Can you work these out from the model? Positions are in its coordinate system, mm. A direction names the side the tool comes from. Give positions to 0.01 mm unless a question says otherwise; leave off trailing zeros. Write each loop counter-clockwise with the first axis right and the second up, starting at its lowest first coordinate (ties: lowest second). Pieces come first, ordered by that corner, then holes.
1. If I drill on probe 1 along X at (y, z) = (20, -157); probe 2 along Y at (x, z) = (256.5, -42.5), over which ranges is the centre line in solid material (lowest first)?
2. Suppose I cut it at C-C (x = 97.5). Please give me the cut outline in (y, z), and give its area (3 significant figures).
3. On a 3-axis mill with a long thin cutter (end or side, diameter ignored), from which of +Z, -Z, +X, -X, +Y, -Y can I reach the whole of each face in a straight line? I mean faces 4 (the flat face through (-350, 30, 4)), 5 (the flat face through (-353.062, 23, 4)). Say none if no direction works.
4. Suppose I cut it at A-A (y = 12). Please give me the cut outline in (x, z).
5. I'm going to push a flat-ended pin straight in: pin 1 (8 mm diameter, centred on x = -246.5, z = -83, fed in from +Y). Where does the tip first touch, or does it pass through?
6. Thinking about a two-plate mould opening in X: for faces 1 (the flat face through (-5, -15, 4)), 2 (the flat face through (353.062, 22, 4)), 3 (the flat face through (5, 0, 4)), which applies, pulls with the +X half, pulls with the -X half, needs draft (parallel to the pull), parting line crosses it, or undercut?
7. Suppose I cut it at B-B (z = -174). Please give me the cut outline in (x, y), and give its area (3 significant figures).
```python
from build123d import *

# Parameters (mm, degrees)
SALIENTE_EXTRUIR1_DEPTH = 300


with BuildPart() as part:
    # Croquis1 → Saliente-Extruir1 (new, symmetric)
    with BuildSketch(Plane.XY):
        Polygon((0, -15), (0, 0), (-350, 0), (-350, 60), (-353.0625, 60), (-353.0625, -15), align=None)
        Polygon((350, 60), (350, 0), (0, 0), (0, -15), (353.0625, -15), (353.0625, 60), align=None)
    extrude(amount=SALIENTE_EXTRUIR1_DEPTH, both=True)


solid = part.part
```
Checks:
1. probe 1: x = -353.06 to -350, 350 to 353.06
1. probe 2: y = -15 to 0
2. outline: (-15, -300) - (0, -300) - (0, 300) - (-15, 300) - close
2. area: 9,000 mm2
3. face 4: +Z, -Z, +Y
3. face 5: +Z, -Z, -X, +Y, -Y
4. outline: (-353.06, -300) - (-350, -300) - (-350, 300) - (-353.06, 300) - close; (350, -300) - (353.06, -300) - (353.06, 300) - (350, 300) - close
5. pin 1: stops at y = 0
6. face 1: needs draft
6. face 2: pulls with the +X half
6. face 3: undercut
7. outline: (-353.06, -15) - (353.06, -15) - (353.06, 60) - (350, 60) - (350, 0) - (-350, 0) - (-350, 60) - (-353.06, 60) - close
7. area: 11,000 mm2
